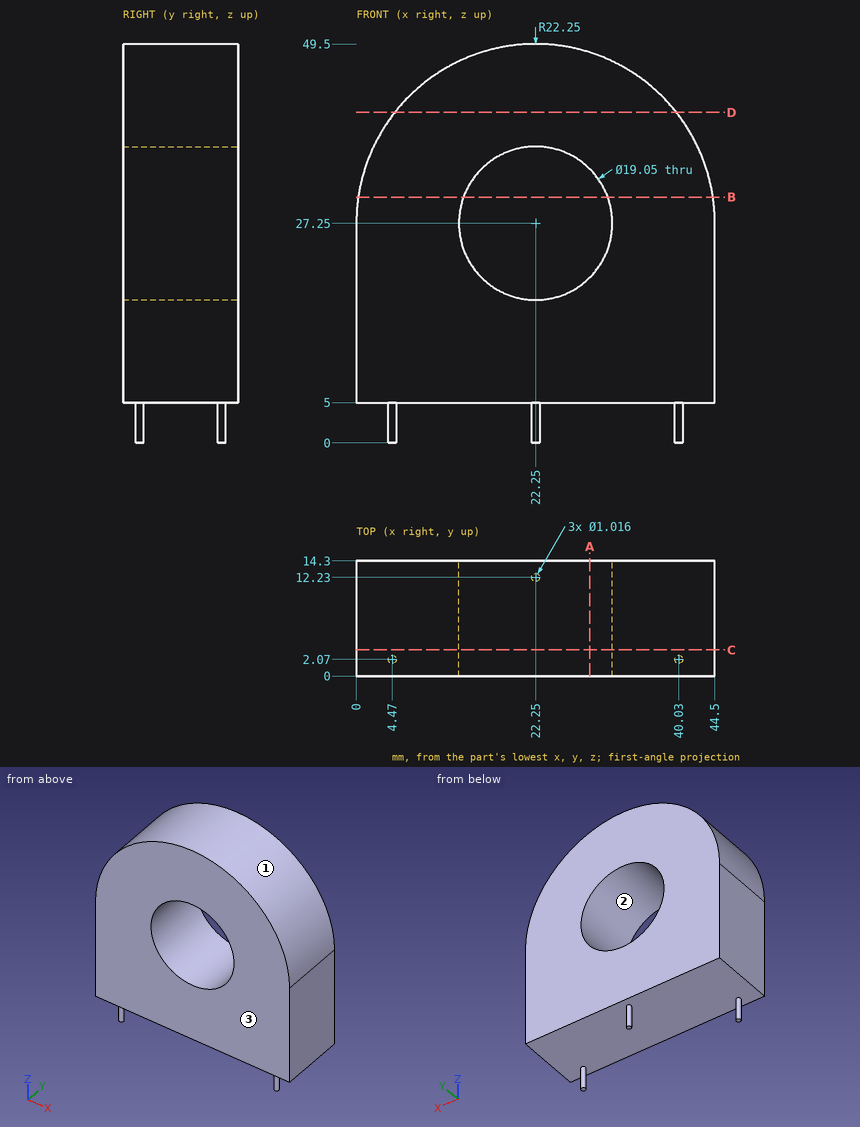
Design review of the part shown in the three views and the two pictorial views. Dimensions are in mm from the part's minimum x, y and z. Round coordinates to 2 decimals unless told otherwise and drop trailing zeros. Order: outer loops, then holes, each group sorted by start corner. A loop starts at its lowest first (then second) coordinate and runs counter-clockwise, first axis right, second up. Notation, with made-up numbers: M -20,86.5 L 39,86.5 A29 ccw 39,107.5 Z; hole C 85.25,28.5 d11. An arc over 180 degrees is marked long. Put each result on its own line as item: value.
Q1. Insertion check: pin 1 Ø6 at (x, y) = (5.5, 10.5) entering from +Z; pin 2 Ø3 at (x, y) = (6, 7.5) entering from +Z; pin 3 Ø1.5 at (x, y) = (32, 4) entering from +Z. Each pin has a flat end and moves straight along its axis. Give the tip position at first contact, or say it passes through.
Reported:
pin 1: z = 44.74
pin 2: z = 43.91
pin 3: z = 47.6
Q2. Consider section C-C (y = 3.25). State the section outline as (x, z) points (3 decimals), and give its area (3 significant figures).
Reported:
outline: M 0,5 L 44.5,5 L 44.5,27.25 A22.25 ccw 0,27.25 Z; hole C 22.25,27.25 d19.05
area: 1,480 mm²
Q3. To check wall thickness, follow line 1 (Z direction, x = 22.25, y = 8.25) (3 decimals); line 2 (X direction, y = 9.5, z = 36); line 3 (X direction, y = 2.5, z = 4). State the ranges of each line that lie inside material, in increasing order.
Reported:
line 1: 5 to 17.725, 36.775 to 49.5
line 2: 1.79 to 18.49, 26.01 to 42.71
line 3: 4.2 to 4.74, 39.76 to 40.3
Q4. Draft analysis for pull direction Z (two halves, no side actions). For the marked faces 1, 2 and 3, state which applies: released by +Z, released by -Z, zero draft, split by the parting line, or undercut.
Reported:
face 1: released by +Z
face 2: undercut
face 3: zero draft
Q5. Consider section B-B (z = 30.5). State the section outline as (x, y) points.
Reported:
outline: M 0.24,0 L 13.3,0 L 13.3,14.3 L 0.24,14.3 Z; M 31.2,0 L 44.26,0 L 44.26,14.3 L 31.2,14.3 Z
Q6. Consider section D-D (z = 41). State the section outline as (x, y) points, and give its area (3 significant figures).
Reported:
outline: M 4.76,0 L 39.74,0 L 39.74,14.3 L 4.76,14.3 Z
area: 500 mm²
Q7. Consider section A-A (x = 29). State the section outline as (y, z) points, and give its area (3 significant figures).
Reported:
outline: M 0,5 L 14.3,5 L 14.3,20.53 L 0,20.53 Z; M 0,33.97 L 14.3,33.97 L 14.3,48.45 L 0,48.45 Z
area: 429 mm²
